Part print with two shaded views. Sizes in mm from the minimum x, y, z corner. Give positions to 0.01 mm unless a question says otherwise; leave off trailing zeros. Write each question's results on one line, items separated by ' | '. Start each with the question number.
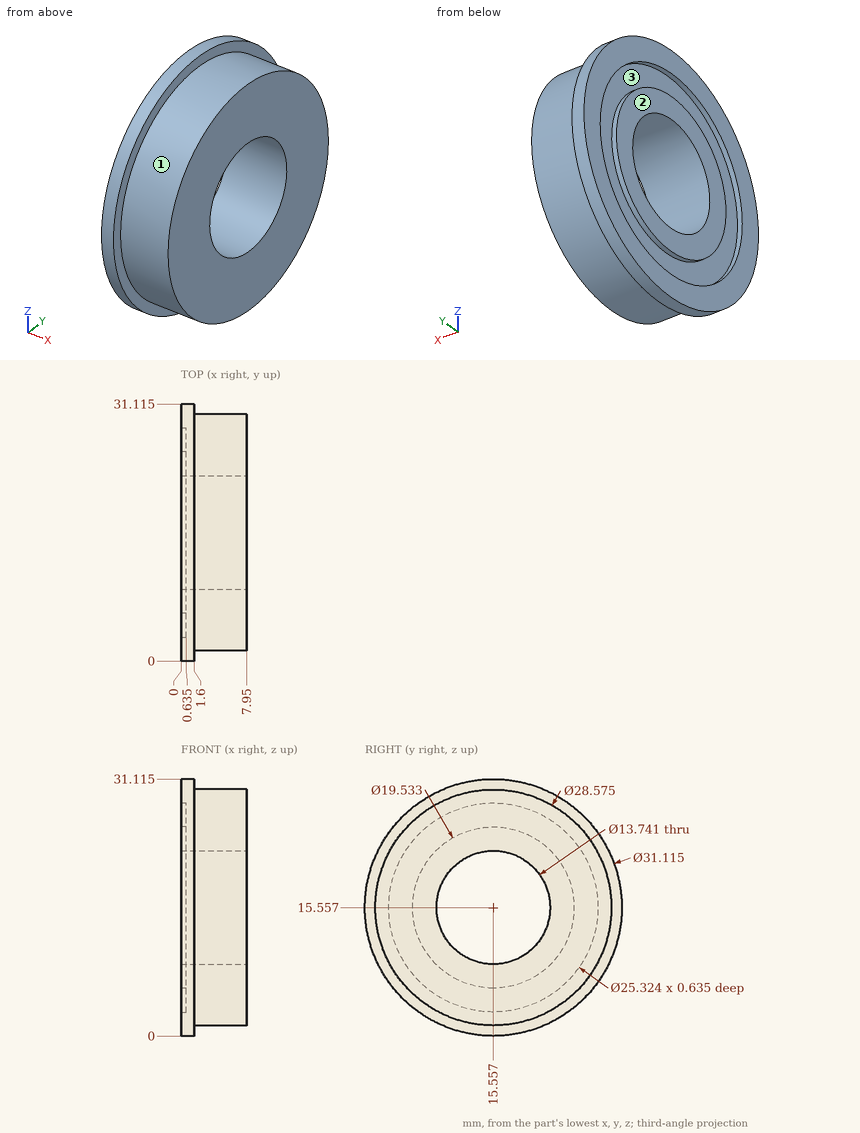
(1) Drop flat-ended pins along their axis: P1, Ø1.5, axis at x = 1.5, y = 13, coming from the -Z side (1 decimal); P2, Ø3, axis at x = 2, y = 10.5, coming from the -Z side (1 decimal); P3, Ø18, axis at y = 15.56, z = 15.56, coming from the +X side. Give the stop position or say it passes through.
(2) Probe L1, parallel to Z at x = 3.25, y = 15.5 (1 decimal); L2, parallel to X at y = 8, z = 2; L3, parallel to Y at x = 5.5, z = 12 (1 decimal). List the from-to ranges inside material, lowest first.
(3) Pull direction Z, two halves, no side cores. Call the marked faces 1, 2 and 3: +Z half, -Z half, draft (parallel to the pull), parting line (faces both ways), or undercut.
Taken from the geometry:
1) P1: stops at z = 0.1 | P2: stops at z = 0.4 | P3: stops at x = 7.95
2) L1: z = 1.3 to 8.7, 22.4 to 29.8 | L2: x = 0 to 1.6 | L3: y = 1.7 to 9.7, 21.4 to 29.4
3) face 1: parting line | face 2: draft | face 3: undercut
